```python
from build123d import *

# Parameters (mm, degrees)
SKETCH1_W            = 355.6
SKETCH1_H            = 50.8
SKETCH1_R            = 2.286
SKETCH1_R_2          = 11.1125
BOTTOM_2_DEPTH       = 3.175
CUT_EXTRUDE1_DEPTH   = 360.224276219
FILLET1_R            = 12.7
BOTTOM_CUTOUT_DEPTH  = 360.224276219
SKETCH5_R            = 11.1125
UPPER_TRIANGLE_DEPTH = 3.175
SKETCH6_R            = 2.286
GEARBOX_HOLES_DEPTH  = 421.704153444
SKETCH7_R            = 2.286
CUT_EXTRUDE4_DEPTH   = 421.704153444
SKETCH8_R            = 2.286
SKETCH8_W            = 22.86
SKETCH8_H            = 22.86
SKETCH8_W_2          = 33.02
SKETCH8_H_2          = 85.725
CUT_EXTRUDE5_DEPTH   = 421.704153444
SKETCH9_R            = 2.286
CUT_EXTRUDE6_DEPTH   = 421.704153444
FILLET2_R            = 6.35
FILLET3_R            = 6.35
SKETCH16_R           = 2.286
CUT_EXTRUDE12_DEPTH  = 421.704153444
FILLET11_R           = 16.51
SKETCH19_R           = 2.54
SKETCH19_R_2         = 2.286
CUT_EXTRUDE14_DEPTH  = 421.704153444
FILLET7_R            = 381
FILLET8_R            = 6.35
SKETCH12_R           = 2.286
CUT_EXTRUDE8_DEPTH   = 421.704153444


with BuildPart() as part:
    # Sketch1 → Bottom 2" (new body)
    with BuildSketch(Plane.XY):
        with Locations((-177.8, 25.4)):
            Rectangle(SKETCH1_W, SKETCH1_H)
        with Locations((-41.91, 6.35)):
            Circle(SKETCH1_R, mode=Mode.SUBTRACT)
        with Locations((-292.735, 6.35)):
            Circle(SKETCH1_R, mode=Mode.SUBTRACT)
        with Locations((-205.74, 19.05)):
            Circle(SKETCH1_R, mode=Mode.SUBTRACT)
        with Locations((-167.3225, 34.29)):
            Circle(SKETCH1_R_2, mode=Mode.SUBTRACT)
        with Locations((-250.085181934, 18.50662125)):
            Circle(SKETCH1_R, mode=Mode.SUBTRACT)
        with Locations((-84.559818066, 18.50662125)):
            Circle(SKETCH1_R, mode=Mode.SUBTRACT)
        with Locations((-128.905, 19.05)):
            Circle(SKETCH1_R, mode=Mode.SUBTRACT)
        with Locations((-338.41529526, 28.575)):
            Circle(SKETCH1_R, mode=Mode.SUBTRACT)
    extrude(amount=BOTTOM_2_DEPTH)

    # Sketch2 → Cut-Extrude1 (cut, through all)
    with BuildSketch(Plane.XY.offset(3.175)):
        Polygon((-384.175, 50.8), (-320.675, 0), (-384.175, 0), align=None)
    extrude(amount=-CUT_EXTRUDE1_DEPTH, mode=Mode.SUBTRACT)

    # Fillet1
    fillet1_edges = [part.edges().sort_by_distance(p)[0] for p in [
        (-355.6, 27.94, 1.5875),
        (-320.675, 0, 1.5875),
    ]]
    fillet(fillet1_edges, radius=FILLET1_R)

    # Sketch3 → Bottom Cutout (cut, through all)
    with BuildSketch(Plane.XY.offset(3.175)):
        Polygon((-256.54, 0), (-205.74, 6.35), (-128.905, 6.35), (-78.105, 0), align=None)
    extrude(amount=-BOTTOM_CUTOUT_DEPTH, mode=Mode.SUBTRACT)

    # Sketch5 → Upper Triangle (add)
    with BuildSketch(Plane.XY.offset(3.175)):
        Polygon((15.24, 50.8), (15.24, 224.79), (-22.86, 224.79), (-355.6, 50.8), align=None)
        with Locations((-3.81, 205.74)):
            Circle(SKETCH5_R, mode=Mode.SUBTRACT)
    extrude(amount=-UPPER_TRIANGLE_DEPTH)

    # Sketch6 → Gearbox Holes (cut, through all)
    with BuildSketch(Plane.XY.offset(3.175)):
        with Locations((-110.1725, 46.99)):
            Circle(SKETCH6_R)
        with Locations((-167.3225, 11.43)):
            Circle(SKETCH6_R)
        with Locations((-224.4725, 46.99)):
            Circle(SKETCH6_R)
    extrude(amount=-GEARBOX_HOLES_DEPTH, mode=Mode.SUBTRACT)

    # Sketch7 → Cut-Extrude4 (cut, through all)
    with BuildSketch(Plane.XY.offset(3.175)):
        with Locations((-25.4, 60.96)):
            Circle(SKETCH7_R)
    extrude(amount=-CUT_EXTRUDE4_DEPTH, mode=Mode.SUBTRACT)

    # Sketch8 → Cut-Extrude5 (cut, through all)
    with BuildSketch(Plane.XY.offset(3.175)):
        with Locations((7.62, 142.875)):
            Circle(SKETCH8_R)
        with Locations((-157.48, 138.632493002)):
            Circle(SKETCH8_R)
        with Locations((-10.16, 160.655)):
            Rectangle(SKETCH8_W, SKETCH8_H)
        with Locations((-1.27, 93.6625)):
            Rectangle(SKETCH8_W_2, SKETCH8_H_2)
        Polygon((-43.18, 185.501736062), (-43.18, 57.15), (-288.640984293, 57.15), align=None)
    extrude(amount=-CUT_EXTRUDE5_DEPTH, mode=Mode.SUBTRACT)

    # Sketch9 → Cut-Extrude6 (cut, through all)
    with BuildSketch(Plane(origin=(0, 0, 0), x_dir=(-1, 0, 0), z_dir=(0, 0, -1))):
        with Locations((10.16, 46.99)):
            Circle(SKETCH9_R)
        with Locations((72.39, 46.99)):
            Circle(SKETCH9_R)
    extrude(amount=-CUT_EXTRUDE6_DEPTH, mode=Mode.SUBTRACT)

    # Fillet2
    fillet2_edges = [part.edges().sort_by_distance(p)[0] for p in [
        (-43.18, 185.501736062, 1.5875),
        (-43.18, 57.15, 1.5875),
        (15.24, 136.525, 1.5875),
        (-17.78, 136.525, 1.5875),
        (-355.6, 50.8, 1.5875),
        (15.24, 224.79, 1.5875),
        (-22.86, 224.79, 1.5875),
    ]]
    fillet(fillet2_edges, radius=FILLET2_R)

    # Fillet3
    fillet3_edges = [part.edges().sort_by_distance(p)[0] for p in [
        (1.27, 172.085, 1.5875),
        (1.27, 149.225, 1.5875),
        (-21.59, 149.225, 1.5875),
        (-21.59, 172.085, 1.5875),
    ]]
    fillet(fillet3_edges, radius=FILLET3_R)

    # Sketch16 → Cut-Extrude12 (cut, through all)
    with BuildSketch(Plane.XY.offset(3.175)):
        with Locations((-262.255, 46.99)):
            Circle(SKETCH16_R)
    extrude(amount=-CUT_EXTRUDE12_DEPTH, mode=Mode.SUBTRACT)

    # Fillet11
    fillet11_edges = [part.edges().sort_by_distance(p)[0] for p in [
        (-288.640984293, 57.15, 1.5875),
    ]]
    fillet(fillet11_edges, radius=FILLET11_R)

    # Sketch19 → Cut-Extrude14 (cut, through all)
    with BuildSketch(Plane.XY.offset(3.175)):
        with Locations((-275.59, 85.09)):
            Circle(SKETCH19_R)
        with Locations((-243.84, 80.01)):
            Circle(SKETCH19_R_2)
    extrude(amount=-CUT_EXTRUDE14_DEPTH, mode=Mode.SUBTRACT)

    # Fillet7
    fillet7_edges = [part.edges().sort_by_distance(p)[0] for p in [
        (-78.105, 0, 1.5875),
        (-256.54, 0, 1.5875),
        (-205.74, 6.35, 1.5875),
        (-128.905, 6.35, 1.5875),
    ]]
    fillet(fillet7_edges, radius=FILLET7_R)

    # Fillet8
    fillet8_edges = [part.edges().sort_by_distance(p)[0] for p in [
        (-17.78, 50.8, 1.5875),
        (0, 50.8, 1.5875),
        (0, 0, 1.5875),
    ]]
    fillet(fillet8_edges, radius=FILLET8_R)

    # Sketch12 → Cut-Extrude8 (cut, through all)
    with BuildSketch(Plane.XY.offset(3.175)):
        with Locations((-336.804, 43.18)):
            Circle(SKETCH12_R)
        with Locations((-273.304, 43.18)):
            Circle(SKETCH12_R)
    extrude(amount=-CUT_EXTRUDE8_DEPTH, mode=Mode.SUBTRACT)


solid = part.part
```
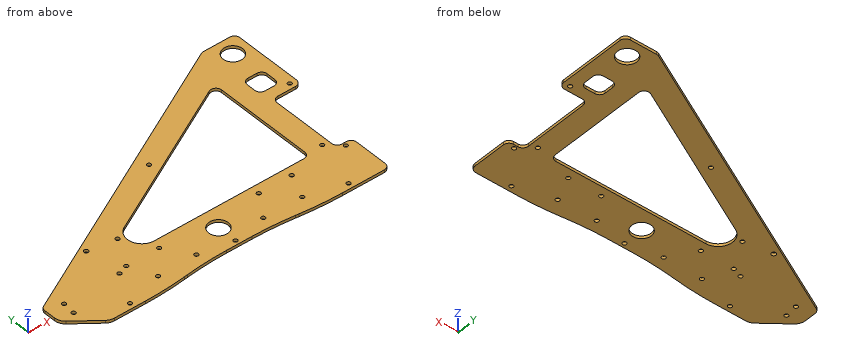
Could you check a few things on this model? Use its own coordinates, in mm. Round coordinates to 2 decimals unless told otherwise and drop trailing zeros. Loops run counter-clockwise (first coordinate to the right, second up) from the corner with the lowest first, then second, coordinate; pieces in that order, holes last. Notation, with made-up numbers: M 23,-39 L 65,-39 A14 cw 65,-16 Z; hole C 36,-6 d11. An arc over 180 degrees is marked long. Write item = value, one per line.
1. I need wall thicknesses on probe 1 along X at (y, z) = (81.5, 1.6); probe 2 along X at (y, z) = (171, 2.15); probe 3 along X at (y, z) = (19, 1.3) (3 decimals). Which ranges of each line are inside material? Lowest first, please.
Results below:
probe_1 = -296.89 to -245.57, -242.11 to -235.97, -43.18 to -17.78
probe_2 = -125.73 to -70.91, -43.18 to -18.79, -1.53 to 15.24
probe_3 = -344.425 to -252.317, -247.853 to -208.025, -203.455 to -131.19, -126.62 to -86.792, -82.328 to 0
2. I want a section at A-A, the plane y = 205.74. Write out the boundary of the cut face in (x, z) (1 decimal), and give its area (3 significant figures).
Results below:
outline = M -59.3,0 L -14.9,0 L -14.9,3.2 L -59.3,3.2 Z; M 7.3,0 L 15.2,0 L 15.2,3.2 L 7.3,3.2 Z
area = 166 mm²
3. I want a section at C-C, the plane z = 0.85. Count the separate pieces of the cut face and the enclosed holes in it, and give its area (3 significant figures).
Results below:
separate_pieces = 1
enclosed_holes = 24
area = 32,900 mm²
4. I want a section at B-B, the plane x = -306. Write out the boundary of the cut face in (y, z) (3 decimals), and give its area (3 significant figures).
Results below:
outline = M 0,0 L 76.736,0 L 76.736,3.175 L 0,3.175 Z
area = 244 mm²
5. Will these pins go through, and if not, where does the flat tip stop? P1, Ø20, axis at x = -167.32, y = 34.29, coming from the -Z side; P2, Ø1.6, axis at x = -3.5, z = 2, coming from the -Y side.
Results below:
P1 = through
P2 = 0.34
